Read the model definition and answer for the solid it produces. Units are mm, in the model's axes. Round coordinates to 2 decimals unless told otherwise and drop trailing zeros. Loops run counter-clockwise (first coordinate to the right, second up) from the corner with the lowest first, then second, coordinate; pieces in that order, holes last. Notation, with made-up numbers: M 59.25,42 L 75.25,42 A29 cw 75.25,66 Z; hole C -36,30 d1. An arc over 180 degrees is marked long. Write each question's results on one line, items separated by ' | '.
```python
from build123d import *

# Parameters (mm, degrees)
F1_DEPTH = 520.7
F3_DEPTH = 50.8


with BuildPart() as f1:
    # F0 (on Right) → F1 (new body)
    with BuildSketch(Plane.YZ):
        with BuildLine():
            Line((-31.75, 0), (0, 0))
            Line((0, 0), (0, 31.75))
            Line((0, 31.75), (-6.35, 31.75))
            ThreePointArc((-6.35, 31.75), (-13.789488, 13.789488), (-31.75, 6.35))
            Line((-31.75, 6.35), (-31.75, 0))
        make_face()
    extrude(amount=F1_DEPTH)

    # F2 (on face) → F3 (cut)
    with BuildSketch(Plane(origin=(0, 0, 0), x_dir=(-1, 0, 0), z_dir=(0, 1, 0))):
        Polygon((0, 0), (0, 31.75), (-31.75, 0), align=None)
        Polygon((-488.95, 0), (-520.7, 31.75), (-520.7, 0), align=None)
    extrude(amount=-F3_DEPTH, mode=Mode.SUBTRACT)


solid = f1.part
```
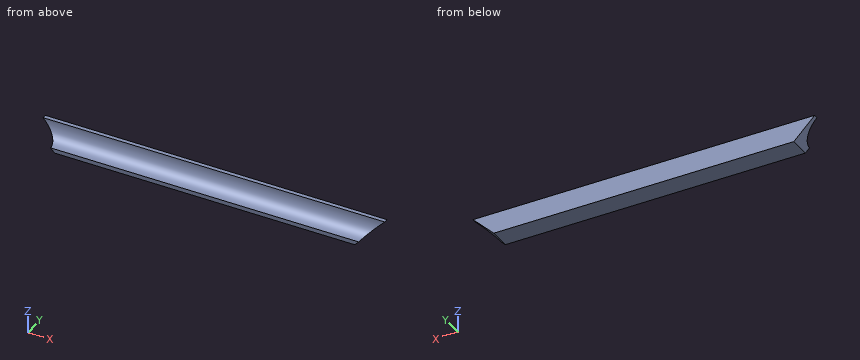
1. Find the intervals of material crossed by L1, parallel to Y at x = 350, z = 15; L2, parallel to Z at x = 388.5, y = -18; L3, parallel to X at y = -4, z = 19.5, in increasing order.
Completed:
L1: y = -12.66 to 0 | L2: z = 0 to 10.39 | L3: x = 12.25 to 508.45
2. Find section A-A, the plane y = -21.5. Give the vertices of the cut face in (x, z), then the cut area to 3 significant figures.
Completed:
outline: M 23.24,8.51 L 31.75,0 L 488.95,0 L 497.46,8.51 Z | area: 3,960 mm2
3. Find section B-B, the plane x = 288. Give the vertices of the cut face in (y, z), then the cut area to 3 significant figures.
Completed:
outline: M -31.75,0 L 0,0 L 0,31.75 L -6.35,31.75 A25.4 cw -31.75,6.35 Z | area: 501 mm2
4. Find section C-C, the plane z = 21.5. Give the vertices of the cut face in (x, y).
Completed:
outline: M 10.25,-8.51 L 510.45,-8.51 L 510.45,0 L 10.25,0 Z
5. Given P1, Ø5, axis at x = 149, z = 17, coming from the -Y side; P2, Ø8, axis at y = -7, z = 5, coming from the -X side; P3, Ø1.5, axis at x = 181.5, y = -13, coming from the +Z side, each flat-ended and moving along its own axis, determine where each tip first touches the part or whether it passes through.
Completed:
P1: stops at y = -13.11 | P2: stops at x = 22.75 | P3: stops at z = 15.47
